Source: CAD feature listing. Evaluate the final solid. Frame: model axes, mm. Face numbers are marked on the shaded views. A direction names the side the tool comes from. Give positions to 0.01 mm unless a question says otherwise; leave off trailing zeros. Write each loop counter-clockwise with the first axis right and the second up, starting at its lowest first coordinate (ties: lowest second). Pieces come first, ordered by that corner, then holes. Notation, with made-up numbers: M -6.5,84.5 L 39.5,84.5 A17 ccw 39.5,91.5 Z; hole C 1.25,13.25 d9. An arc over 180 degrees is marked long. Use CSV: the item, a comma, the result in double quotes. Start each with the question number.
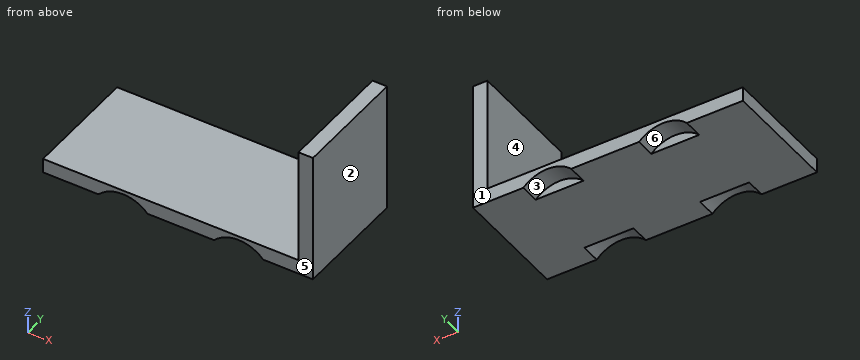
from build123d import *

# Parameters (mm, degrees)
F0_W     = 19.05
F0_H     = 152.4
F1_DEPTH = 76.2
F3_DEPTH = 25.4
F5_DEPTH = 25.4


with BuildPart() as f1:
    # F0 (on Front) → F1 (new body, symmetric)
    with BuildSketch(Plane.XZ):
        Polygon((-177.8, -9.525), (177.8, -9.525), (177.8, 9.525), (158.75, 9.525), (-177.8, 9.525), align=None)
        with Locations((168.275, 85.725)):
            Rectangle(F0_W, F0_H)
    extrude(amount=F1_DEPTH, both=True)

    # F2 (on face) → F3 (cut)
    with BuildSketch(Plane.XZ.offset(76.2)):
        with BuildLine():
            ThreePointArc((-40.0361424247, -9.525), (-72.39, 4.445), (-104.7438575753, -9.525))
            Line((-104.7438575753, -9.525), (-72.39, -9.525))
            Line((-72.39, -9.525), (-40.0361424247, -9.525))
        make_face()
        with BuildLine():
            ThreePointArc((112.3638575753, -9.525), (80.01, 4.445), (47.6561424247, -9.525))
            Line((47.6561424247, -9.525), (80.01, -9.525))
            Line((80.01, -9.525), (112.3638575753, -9.525))
        make_face()
    extrude(amount=-F3_DEPTH, mode=Mode.SUBTRACT)

    # F4 (on face) → F5 (cut)
    with BuildSketch(Plane(origin=(0, 76.2, 0), x_dir=(-1, 0, 0), z_dir=(0, 1, 0))):
        with BuildLine():
            ThreePointArc((-48.4944535083, -9.525), (-80.0064127753, 3.5753760285), (-111.5183720423, -9.525))
            Line((-111.5183720423, -9.525), (-48.4944535083, -9.525))
        make_face()
        with BuildLine():
            ThreePointArc((103.9055464917, -9.525), (72.3935872247, 3.5753760285), (40.8816279577, -9.525))
            Line((40.8816279577, -9.525), (103.9055464917, -9.525))
        make_face()
    extrude(amount=-F5_DEPTH, mode=Mode.SUBTRACT)


solid = f1.part
Item 1: Section B-B (z = 55). Return the cut outline in (x, y), plus the area to 3 significant figures.
Item 2: Contact query for flat-ended pins moving along their axis: pin 1 Ø1.5 at (y, z) = (-0.5, 125.5) entering from -X; pin 2 Ø5 at (x, y) = (94.5, 5) entering from +Z (3 decimals); pin 3 Ø7 at (x, z) = (76, -5.5) entering from -Y. Output: stop coordinate, or through.
Item 3: Section C-C (y = -60). Return the cut outline in (x, z) (3 decimals).
Item 4: Section A-A (y = 58.5). Return the cut outline in (x, z) (3 decimals), plus the area to 3 significant figures.
Item 5: Set-up query: the marked faces 4, 5 and 6. Return all of +Z, -Z, +X, -X, +Y, -Y with unobstructed straight access to the full face (end or side cutting, diameter ignored); none if empty.
Item 6: Section D-D (x = -10.5). Return the cut outline in (y, z) (3 decimals), plus the area to 3 significant figures.
Item 7: Pull-direction query (X, two-part tool) for the marked faces 1, 2 and 3; classes: released by +X, released by -X, zero draft, split by the parting line, or undercut.
Item 8: Material intervals for probe 1 along X at (y, z) = (-57, 33); probe 2 along Z at (x, y) = (129.5, 1.5) (3 decimals), sorted ascending.
Output values:
1,outline,"M 158.75,-76.2 L 177.8,-76.2 L 177.8,76.2 L 158.75,76.2 Z"
1,area,"2,900 mm2"
2,pin 1,"stops at x = 158.75"
2,pin 2,"stops at z = 9.525"
2,pin 3,"stops at y = -50.8"
3,outline,"M -177.8,-9.525 L -104.744,-9.525 A44.45 cw -40.036,-9.525 L 47.656,-9.525 A44.45 cw 112.364,-9.525 L 177.8,-9.525 L 177.8,161.925 L 158.75,161.925 L 158.75,9.525 L -177.8,9.525 Z"
4,outline,"M -177.8,-9.525 L -103.906,-9.525 A44.45 cw -40.882,-9.525 L 48.494,-9.525 A44.45 cw 111.518,-9.525 L 177.8,-9.525 L 177.8,161.925 L 158.75,161.925 L 158.75,9.525 L -177.8,9.525 Z"
4,area,"8,540 mm2"
5,face 4,"+Z, -X, +Y, -Y"
5,face 5,"+Z, -Z, +X, -X, -Y"
5,face 6,"-Z, +Y"
6,outline,"M -76.2,-9.525 L 76.2,-9.525 L 76.2,9.525 L -76.2,9.525 Z"
6,area,"2,900 mm2"
7,face 1,"zero draft"
7,face 2,"released by +X"
7,face 3,"undercut"
8,probe 1,"x = 158.75 to 177.8"
8,probe 2,"z = -9.525 to 9.525"
